```python
from build123d import *

# Parameters (mm, degrees)
SKETCH1_W                   = 31.75
SKETCH1_H                   = 12.7
BOSS_EXTRUDE1_DEPTH         = 25.4
F_1_4_20_TAPPED_HOLE1_D     = 5.1054
F_1_4_20_TAPPED_HOLE1_DEPTH = 16.51
F_1_4_20_TAPPED_HOLE1_TIP   = 1.533816902


with BuildPart() as part:
    # Sketch1 → Boss-Extrude1 (new body)
    with BuildSketch(Plane.XY):
        Rectangle(SKETCH1_W, SKETCH1_H)
    extrude(amount=BOSS_EXTRUDE1_DEPTH)

    # 1/4-20 Tapped Hole1
    with Locations(Plane.XY.offset(25.4)):
        with Locations((-9.525, 0), (9.525, 0)):
            Hole(F_1_4_20_TAPPED_HOLE1_D / 2, depth=F_1_4_20_TAPPED_HOLE1_DEPTH)
            with Locations((0, 0, -(F_1_4_20_TAPPED_HOLE1_DEPTH + F_1_4_20_TAPPED_HOLE1_TIP / 2))):  # 118° drill point
                Cone(0, F_1_4_20_TAPPED_HOLE1_D / 2, F_1_4_20_TAPPED_HOLE1_TIP, mode=Mode.SUBTRACT)


solid = part.part
```
Geometry: final body of the model. Coordinates: model frame, mm. A direction names the side the tool comes from. Round coordinates to 2 decimals unless told otherwise and drop trailing zeros. Loops run counter-clockwise (first coordinate to the right, second up) from the corner with the lowest first, then second, coordinate; pieces in that order, holes last.
Item 1: Line query: L1, parallel to X at y = 0, z = 12.5 (3 decimals); L2, parallel to X at y = 1.5, z = 9.25 (1 decimal); L3, parallel to Y at x = 11, z = 22.25. Output: solid intervals per line, ascending.
Checked values:
L1: x = -15.875 to -12.078, -6.972 to 6.972, 12.078 to 15.875
L2: x = -15.9 to -11.6, -7.5 to 7.5, 11.6 to 15.9
L3: y = -6.35 to -2.08, 2.08 to 6.35
Item 2: Mould query, pull axis X, two halves, no side actions, for faces 1 (the conical face through (9.173, -0.27, 7.623)), 2 (the flat face through (15.875, 0, 13)), 3 (the flat face through (-15.875, 0, 13)), 4 (the flat face through (0, -6.35, 13)). Classes: released by +X, released by -X, zero draft, split by the parting line, or undercut.
Checked values:
face 1: undercut
face 2: released by +X
face 3: released by -X
face 4: zero draft
Item 3: Section A-A, the plane z = 9.75. Output: boundary loops of the cut face in (x, y) (3 decimals), plus the area to 3 significant figures.
Checked values:
outline: (-15.875, -6.35) - (15.875, -6.35) - (15.875, 6.35) - (-15.875, 6.35) - close; hole circle Ø5.105 at (-9.525, 0); hole circle Ø5.105 at (9.525, 0)
area: 362 mm2
Item 4: Reachability of faces 5 (the cylindrical face through (-7.644, 1.725, 17.029)), 6 (the flat face through (0, 0, 25.4)) from +Z, -Z, +X, -X, +Y, -Y: full face, straight path, thin tool, end or side. Return the list, or none.
Checked values:
face 5: +Z
face 6: +Z, +X, -X, +Y, -Y
